Source: CAD feature listing. Evaluate the final solid. Frame: model axes, mm. A direction names the side the tool comes from. Round coordinates to 2 decimals unless told otherwise and drop trailing zeros. Order: outer loops, then holes, each group sorted by start corner. A loop starts at its lowest first (then second) coordinate and runs counter-clockwise, first axis right, second up. Notation, with made-up numbers: (60.25, 11) - (104.25, 11) arc R17 ccw to (104.25, 32) - close; hole circle Ø6 at (7.5, -11.5). An arc over 180 degrees is marked (long way). Return JSON: item names as keys, results as strings. Group by question number.
1) Section A-A, the plane y = 4.75. Return loops of the section in (x, z).
2) Access query for faces 1 (the cylindrical face through (12.62, 5.031, -22.657)), 2 (the cylindrical face through (73.43, 14.45, -1.82)). Directions: +Z, -Z, +X, -X, +Y, -Y. A direction counts if a zero-diameter tool reaches every point of the face in a straight line with its end or side. Return the directions, or none.
3) Section B-B, the plane x = 12.1. Return loops of the section in (y, z), plus the area to 3 significant figures.
4) Mould query, pull axis X, two halves, no side actions, for faces 3 (the cylindrical face through (50.92, 24.48, -24.65)), 4 (the cylindrical face through (26.51, 14.447, -1.134)), 5 (the flat face through (100, 11, -24)). Classes: pulls with the +X half, pulls with the -X half, needs draft (parallel to the pull), parting line crosses it, or undercut.
5) Section D-D, the plane z = -11. Return loops of the section in (x, y).
6) Section C-C, the plane y = 20.5. Return loops of the section in (x, z), plus the area to 3 significant figures.
7) Contact query for flat-ended pins moving along their axis: P1, Ø2, axis at y = 16.5, z = -22.5, coming from the -X side; P2, Ø1.4, axis at x = 88.5, z = -25, coming from the -Y side; P3, Ø3, axis at x = 82, z = -19, coming from the +Y side; P4, Ø10, axis at x = 13, z = -19, coming from the +Y side. Output: stop coordinate, or through.
8) Ray query, line 1 (X direction, y = 5, z = -25); line 2 (Y direction, x = 10, z = -16.5); line 3 (Y direction, x = 39, z = -25). Return the intervals inside material, ascending. Write a range as from..to.
Autodesk Inventor part; units mm, degrees
ref_plane "YZ Plane" through (0, 0, 0) normal (1, 0, 0) x (0, 1, 0)
ref_plane "XZ Plane" through (0, 0, 0) normal (0, 1, 0) x (-1, 0, 0)
ref_plane "XY Plane" through (0, 0, 0) normal (0, 0, 1) x (1, 0, 0)
sketch "Sketch1" plane through (0, 0, 0) normal (0, 1, 0) x (-1, 0, 0)
  line L0 (-3, 0) -> (-97, 0)
  line L1 (-100, -3) -> (-100, -47)
  line L2 (-97, -50) -> (-3, -50)
  line L3 (0, -47) -> (0, -3)
  line L4 (0, -50) -> (0, -25)
  line L5 (0, -25) -> (-12.1, -25)
  circle A0 centre (-12.1, -25) radius 2.4
  line L6 (-12.1, -25) -> (-87.8936, -25)
  circle A1 centre (-87.8936, -25) radius 2.4
  arc A2 (0, -3) -> (-3, 0) centre (-3, -3) ccw
  arc A3 (-3, -50) -> (0, -47) centre (-3, -47) ccw
  arc A4 (-97, 0) -> (-100, -3) centre (-97, -3) ccw
  arc A5 (-100, -47) -> (-97, -50) centre (-97, -47) ccw
  point P0 (0, 0)
  point P1 (-100, -50)
  point P2 (-100, 0)
  dimension "d0" = 100
  dimension "d1" = 50
  dimension "d2" = 25
  dimension "d3" = 12.1
  dimension "d4" = 4.8
  dimension "d5" = 75.7936
  dimension "d6" = 4.8
  dimension "d7" = 3
extrude "Extrusion1" add sketch "Sketch1" along normal blind 10
sketch "Sketch2" plane through (0, 10, 0) normal (0, 1, 0) x (1, 0, 0)
  line L0 (2, 0) -> (98, 0)
  line L1 (100, 2) -> (100, 48)
  line L2 (98, 50) -> (2, 50)
  line L3 (0, 48) -> (0, 2)
  arc A0 (98, 0) -> (100, 2) centre (98, 2) ccw
  arc A1 (0, 2) -> (2, 0) centre (2, 2) ccw
  arc A2 (2, 50) -> (0, 48) centre (2, 48) ccw
  arc A3 (100, 48) -> (98, 50) centre (98, 48) ccw
  point P0 (0, 0)
  dimension "d10" = 2
extrude "Extrusion2" add sketch "Sketch2" along normal blind 18.3
sketch "Sketch3" plane through (3, 0, 0) normal (0, 0, 1) x (1, 0, 0)
  point P0 (-3, 0)
sketch "Sketch4" plane through (0, 28.3, 0) normal (0, 1, 0) x (1, 0, 0)
  line L0 (3, 0) -> (97, 0)
  arc A0 (6.1709, 4.1832) -> (50, 0) centre (48.8144, 219.278) ccw
  line L1 (0, 47) -> (0, 3)
  arc A1 (0, 25) -> (6.1709, 4.1832) centre (35.6265, 24.238) ccw
  arc A2 (6.1709, 44.2928) -> (0, 25) centre (35.6265, 24.238) ccw
  line L2 (97, 50) -> (3, 50)
  arc A3 (50, 50) -> (6.1709, 44.2928) centre (53.6635, -149.2845) ccw
  arc A4 (92.3505, 44.2928) -> (50, 50) centre (45.5073, -143.3251) ccw
  line L3 (100, 3) -> (100, 47)
  arc A5 (100, 25) -> (92.3505, 44.2928) centre (73.1068, 25.5) ccw
  arc A6 (92.3505, 6.7071) -> (100, 25) centre (77.2233, 23.7786) ccw
  arc A7 (50, 0) -> (92.3505, 6.7071) centre (52.254, 122.8285) ccw
  point P0 (0, 0)
extrude "Extrusion3" cut sketch "Sketch4" against normal blind 28.1 keep common part
sketch "Sketch5" plane through (47.6287, 28.3, 0) normal (0, 0, 1) x (1, 0, 0)
  line L0 (0, 0) -> (6.8792, 0)
  line L1 (3.4396, 0) -> (-6.5604, 0)
  line L2 (3.4396, 0) -> (13.4396, 0)
  line L3 (6.8792, 0) -> (44.7218, 0)
  arc A0 (-6.5604, 0) -> (13.4396, 0) centre (3.4396, 11.1803) ccw
  point P0 (-47.6287, -28.3)
  dimension "d15" = 10
  dimension "d16" = 10
  dimension "d17" = 15
extrude "Extrusion4" cut sketch "Sketch5" against normal blind 50
sketch "Sketch6" plane through (47.6287, 0.2, 0) normal (0, 0, 1) x (1, 0, 0)
  arc A0 (-6.5604, 28.1) -> (-46.762, 22.2881) centre (-6.5604, -113.8444) ccw
  arc A1 (52.1024, 22.2904) -> (13.4396, 28.1) centre (13.4396, -103.4557) ccw
  line L0 (52.1024, 22.2904) -> (52.3713, 28.1)
  line L1 (52.3713, 28.1) -> (13.4396, 28.1)
  line L2 (-6.5604, 28.1) -> (-47.6287, 28.1)
  line L3 (-47.6287, 28.1) -> (-46.762, 22.2881)
  point P0 (-47.6287, -0.2)
extrude "Extrusion5" cut sketch "Sketch6" against normal blind 50
sketch "Sketch7" plane through (47.6287, 0.2, 0) normal (0, 0, 1) x (1, 0, 0)
  line L0 (-47.6287, 28.1) -> (-47.6287, 0)
  arc A0 (-46.762, 22.2881) -> (-47.6287, 21.9584) centre (-45.4512, 17.5372) ccw
  line L1 (-47.6287, 21.9584) -> (-47.6287, 28.1)
  line L2 (-46.762, 22.2881) -> (-47.6287, 28.1)
  point P0 (-47.6287, -0.2)
extrude "Extrusion6" cut sketch "Sketch7" against normal blind 50
sketch "Sketch8" plane through (47.6287, 0.2, 0) normal (0, 0, 1) x (1, 0, 0)
  line L0 (52.3713, 28.1) -> (52.3713, 0)
  line L1 (52.1024, 22.2904) -> (52.3713, 28.1)
  arc A0 (52.3713, 22.1965) -> (52.1024, 22.2904) centre (49.9324, 15.6487) ccw
  line L2 (52.1024, 22.2904) -> (52.3713, 28.1)
  line L3 (52.3713, 28.1) -> (52.3713, 22.1965)
  point P0 (-47.6287, -0.2)
extrude "Extrusion7" cut sketch "Sketch8" against normal blind 50
properties part number "SSOK"
Geometry check:
{
 "1": {"outline": "(0, -25) arc R35.63 ccw to (6.17, -44.29) arc R199.32 ccw to (50, -50) arc R193.38 ccw to (92.35, -44.29) arc R26.9 ccw to (100, -26) - (100, -22.56) arc R22.81 ccw to (92.35, -6.71) arc R122.85 ccw to (54.51, 0) - (47.63, 0) arc R219.28 ccw to (6.17, -4.18) arc R35.63 ccw to (0, -23.48) - close; hole circle Ø4.8 at (12.1, -25); hole circle Ø4.8 at (87.89, -25)"},
 "2": {"face 1": "-Y", "face 2": "+Z, +X, +Y, -Y"},
 "3": {"outline": "(0.2, -45.65) - (25.31, -45.65) - (25.31, -3.09) - (0.2, -3.09) - (0.2, -22.6) - (10, -22.6) - (10, -27.4) - (0.2, -27.4) - close", "area": "1,020 mm2"},
 "4": {"face 3": "undercut", "face 4": "pulls with the -X half", "face 5": "pulls with the +X half"},
 "5": {"outline": "(2.54, 0.2) - (96.12, 0.2) - (96.12, 23.55) arc R131.56 ccw to (61.07, 28.3) arc R15 cw to (41.07, 28.3) arc R141.95 ccw to (2.54, 22.97) - close"},
 "6": {"outline": "(0, -25) arc R35.63 ccw to (6.17, -44.29) arc R199.32 ccw to (50, -50) arc R193.38 ccw to (92.35, -44.29) arc R26.9 ccw to (100, -26) - (100, -22.56) arc R22.81 ccw to (92.35, -6.71) arc R122.85 ccw to (54.51, 0) - (47.63, 0) arc R219.28 ccw to (6.17, -4.18) arc R35.63 ccw to (0, -23.48) - close", "area": "4,360 mm2"},
 "7": {"P1": "x = 0", "P2": "y = 10", "P3": "y = 26.86", "P4": "y = 26.41"},
 "8": {"line 1": "0..9.7, 14.5..85.49, 90.29..100", "line 2": "0.2..24.86", "line 3": "0.2..28.28"}
}
